from build123d import *

# Parameters (mm, degrees)
F1_DEPTH = 10
F2_R     = 1.9
F3_DEPTH = 4.5


with BuildPart() as f1:
    # F0 (on Right) → F1 (new body)
    with BuildSketch(Plane.YZ):
        Polygon((-10, 0), (0, 0), (0, 165), (-5, 165), (-5, 175), (-10, 175), align=None)
    extrude(amount=F1_DEPTH)

    # F2 (on face) → F3 (cut)
    with BuildSketch(Plane(origin=(0, -5, 0), x_dir=(-1, 0, 0), z_dir=(0, 1, 0))):
        with Locations((-5, 170)):
            Circle(F2_R)
    extrude(amount=-F3_DEPTH, mode=Mode.SUBTRACT)

    # F4: F1 across plane


with BuildPart() as f1_1:
    add(f1.part)
    add(f1.part.mirror(Plane.XY))


solid = f1_1.part
Check sheet for the modelled part. Datum: model origin and axes. Units: mm. A direction names the side the tool comes from. Give positions to 0.01 mm unless a question says otherwise; leave off trailing zeros. Write each loop counter-clockwise with the first axis right and the second up, starting at its lowest first coordinate (ties: lowest second). Pieces come first, ordered by that corner, then holes. Notation, with made-up numbers: (-8, 57) -> (11, 57) arc R11 ccw to (11, 62) -> close; hole circle Ø4 at (-15.5, 88.25). An arc over 180 degrees is marked (long way). Write item = value, one per line.
Item 1: Tool access check on faces 1 (the flat face through (4.9, -5, -167.7)), 2 (the flat face through (4.9, -5, 167.7)), 3 (the flat face through (5, -10, -2)). Record the directions out of +Z, -Z, +X, -X, +Y, -Y that give a thin tool (end or side, any length) a straight path to the whole face; none if there is none.
Output:
face_1 = -Z, +X, -X, +Y
face_2 = +Z, +X, -X, +Y
face_3 = +Z, -Z, +X, -X, -Y
Item 2: Sectioned sample at A-A on x = 5. Record the boundary of the cut face in (y, z), and give its area (3 significant figures).
Output:
outline = (-10, -175) -> (-5, -175) -> (-5, -171.9) -> (-9.5, -171.9) -> (-9.5, -168.1) -> (-5, -168.1) -> (-5, -165) -> (0, -165) -> (0, 165) -> (-5, 165) -> (-5, 168.1) -> (-9.5, 168.1) -> (-9.5, 171.9) -> (-5, 171.9) -> (-5, 175) -> (-10, 175) -> close
area = 3,370 mm^2
Item 3: Scan lines: probe 1 along Z at (x, y) = (5, -6.1); probe 2 along X at (y, z) = (-7.55, -170); probe 3 along Z at (x, y) = (6.75, -3). Record each from-to range of solid material in increasing order. Write a range as from..to.
Output:
probe_1 = -175..-171.9, -168.1..168.1, 171.9..175
probe_2 = 0..3.1, 6.9..10
probe_3 = -165..165
Item 4: Gauge pin test, flat ends, axial feed: pin 1 (1.9 mm diameter, centred on x = 5, z = 169.5, fed in from +Y); pin 2 (2.5 mm diameter, centred on x = 4, y = -2.5, fed in from -Z). Record the tip position at first contact, or that the pin passes through.
Output:
pin_1 = -9.5
pin_2 = -165
